from build123d import *

# Parameters (mm, degrees)
SKETCH1_R                       = 8
BOSS_EXTRUDE1_DEPTH             = 11.65
SKETCH2_R                       = 2.975
BOSS_EXTRUDE2_DEPTH             = 1.82
SKETCH3_R                       = 1.5
BOSS_EXTRUDE3_DEPTH             = 8.15
SKETCH4_W                       = 2.321637354
SKETCH4_H                       = 1.249395682
CUT_EXTRUDE1_DEPTH              = 7
SKETCH5_R                       = 7.75
BOSS_EXTRUDE4_DEPTH             = 27
SKETCH6_W                       = 10.10878331
SKETCH6_H                       = 2.575875473
CUT_EXTRUDE2_DEPTH              = 27
SKETCH7_R                       = 2.325
BOSS_EXTRUDE6_DEPTH             = 2
FILLET1_R                       = 0.2
TAP_DRILL_FOR_M2X0_4_TAP1_D     = 1.6
TAP_DRILL_FOR_M2X0_4_TAP1_DEPTH = 3
TAP_DRILL_FOR_M2X0_4_TAP1_TIP   = 0.480688495


with BuildPart() as part:
    # Sketch1 → Boss-Extrude1 (new body)
    with BuildSketch(Plane.XY):
        Circle(SKETCH1_R)
    extrude(amount=BOSS_EXTRUDE1_DEPTH)

    # Sketch2 → Boss-Extrude2 (add)
    with BuildSketch(Plane(origin=(0, 0, 0), x_dir=(-1, 0, 0), z_dir=(0, 0, -1))):
        with Locations(Location((0, 0, 0), (0, 0, 180))):
            Circle(SKETCH2_R)
    extrude(amount=BOSS_EXTRUDE2_DEPTH)

    # Sketch3 → Boss-Extrude3 (add)
    with BuildSketch(Plane(origin=(0, 0, -1.82), x_dir=(-1, 0, 0), z_dir=(0, 0, -1))):
        Circle(SKETCH3_R)
    extrude(amount=BOSS_EXTRUDE3_DEPTH)

    # Sketch4 → Cut-Extrude1 (cut)
    with BuildSketch(Plane(origin=(0, 0, -9.97), x_dir=(-1, 0, 0), z_dir=(0, 0, -1))):
        with Locations((0, 1.574697841)):
            Rectangle(SKETCH4_W, SKETCH4_H)
    extrude(amount=-CUT_EXTRUDE1_DEPTH, mode=Mode.SUBTRACT)

    # Sketch5 → Boss-Extrude4 (add)
    with BuildSketch(Plane.XY.offset(11.65)):
        Circle(SKETCH5_R)
    extrude(amount=BOSS_EXTRUDE4_DEPTH)

    # Sketch6 → Cut-Extrude2 (cut)
    with BuildSketch(Plane.XY.offset(38.65)):
        with Locations((0, -7.162937736)):
            Rectangle(SKETCH6_W, SKETCH6_H)
    cut_extrude2 = extrude(amount=-CUT_EXTRUDE2_DEPTH, mode=Mode.SUBTRACT)

    # Mirror1: Cut-Extrude2 across plane
    add(cut_extrude2.mirror(Plane.ZX), mode=Mode.SUBTRACT)

    # Sketch7 → Boss-Extrude6 (add)
    with BuildSketch(Plane.XY.offset(38.65)):
        Circle(SKETCH7_R)
    extrude(amount=BOSS_EXTRUDE6_DEPTH)

    # Fillet1
    fillet1_edges = [part.edges().sort_by_distance(p)[0] for p in [
        (-2.325, 0, 40.65),
    ]]
    fillet(fillet1_edges, radius=FILLET1_R)

    # Tap Drill for M2x0.4 Tap1
    with Locations(Plane(origin=(0, 0, 0), x_dir=(-1, 0, 0), z_dir=(0, 0, -1))):
        with Locations((-5.5, 0), (5.5, 0)):
            Hole(TAP_DRILL_FOR_M2X0_4_TAP1_D / 2, depth=TAP_DRILL_FOR_M2X0_4_TAP1_DEPTH)
            with Locations((0, 0, -(TAP_DRILL_FOR_M2X0_4_TAP1_DEPTH + TAP_DRILL_FOR_M2X0_4_TAP1_TIP / 2))):  # 118° drill point
                Cone(0, TAP_DRILL_FOR_M2X0_4_TAP1_D / 2, TAP_DRILL_FOR_M2X0_4_TAP1_TIP, mode=Mode.SUBTRACT)


solid = part.part
Source: CAD feature listing. Evaluate the final solid. Frame: model axes, mm. A direction names the side the tool comes from. Give positions to 0.01 mm unless a question says otherwise; leave off trailing zeros. Order: outer loops, then holes, each group sorted by start corner. A loop starts at its lowest first (then second) coordinate and runs counter-clockwise, first axis right, second up. Notation, with made-up numbers: (-27, -18) -> (-11, -18) arc R14 ccw to (-11, 7) -> close; hole circle Ø1 at (78, -8). An arc over 180 degrees is marked (long way). Write item = value, one per line.
Q1. Cut plane C-C, the plane y = 5. Output: boundary loops of the cut face in (x, z) (3 decimals).
Data:
outline = (-6.245, 0) -> (6.245, 0) -> (6.245, 11.65) -> (5.921, 11.65) -> (5.921, 38.65) -> (-5.921, 38.65) -> (-5.921, 11.65) -> (-6.245, 11.65) -> close
Q2. Pull-direction query (Y, two-part tool) for faces 1 (the face through (5.61, -0.08, 3.4)), 2 (the face through (-0.69, -1.33, -5.84)), 3 (the face through (-5.39, -0.08, 3.4)), 4 (the face through (0, 0, 40.65)); classes: released by +Y, released by -Y, zero draft, split by the parting line, or undercut.
Data:
face_1 = undercut
face_2 = split by the parting line
face_3 = undercut
face_4 = zero draft
Q3. Material intervals for line 1 (X direction, y = 0, z = 2); line 2 (Y direction, x = 2.5, z = 25) (3 decimals); line 3 (Z direction, x = -2, y = -7), sorted ascending. Write a range as from..to.
Data:
line_1 = -8..-6.3, -4.7..4.7, 6.3..8
line_2 = -5.875..5.875
line_3 = 0..11.65
Q4. Cut plane B-B, the plane z = 25. Output: boundary loops of the cut face in (x, y) (3 decimals), and give its area (3 significant figures).
Data:
outline = (-5.054, -5.875) -> (5.054, -5.875) arc R7.75 ccw to (5.054, 5.875) -> (-5.054, 5.875) arc R7.75 ccw to start
area = 163 mm^2
Q5. Cut plane A-A, the plane x = 0. Output: boundary loops of the cut face in (y, z) (3 decimals), and give its area (3 significant figures).
Data:
outline = (-8, 0) -> (-2.975, 0) -> (-2.975, -1.82) -> (-1.5, -1.82) -> (-1.5, -9.97) -> (0.95, -9.97) -> (0.95, -2.97) -> (1.5, -2.97) -> (1.5, -1.82) -> (2.975, -1.82) -> (2.975, 0) -> (8, 0) -> (8, 11.65) -> (5.875, 11.65) -> (5.875, 38.65) -> (2.325, 38.65) -> (2.325, 40.45) arc R0.2 ccw to (2.125, 40.65) -> (-2.125, 40.65) arc R0.2 ccw to (-2.325, 40.45) -> (-2.325, 38.65) -> (-5.875, 38.65) -> (-5.875, 11.65) -> (-8, 11.65) -> close
area = 544 mm^2
Q6. Cut plane D-D, the plane y = -7. Output: boundary loops of the cut face in (x, z).
Data:
outline = (-3.87, 0) -> (3.87, 0) -> (3.87, 11.65) -> (-3.87, 11.65) -> close
Q7. Set-up query: faces 5 (the face through (7.75, -0.09, 24.96)), 6 (the face through (4.7, 0, 1.5)), 7 (the face through (0, -5.875, 25)), 8 (the face through (0, 0.95, -7)). Return all of +Z, -Z, +X, -X, +Y, -Y with unobstructed straight access to the full face (end or side cutting, diameter ignored); none if empty.
Data:
face_5 = +Z, +X
face_6 = -Z
face_7 = +Z, +X, -X, -Y
face_8 = -Z, +X, -X, +Y
Q8. Pin query (flat end, axial travel): pin 1 (6 mm diameter, centred on x = 3.5, y = -2, fed in from +Z); pin 2 (1 mm diameter, centred on y = -5.5, z = 13, fed in from +X); pin 3 (8 mm diameter, centred on x = 5, z = 14, fed in from +Y); pin 4 (2.5 mm diameter, centred on x = -5.5, y = 0, fed in from -Z). Return the tip coordinate at first contact, or that it passes through.
Data:
pin_1 = 40.65
pin_2 = 5.92
pin_3 = 7.8
pin_4 = 0
